Could you check a few things on this model? Use its own coordinates, in mm. Face numbers are marked on the shaded views. A direction names the side the tool comes from. Give positions to 0.01 mm unless a question says otherwise; leave off trailing zeros. Write each loop counter-clockwise with the first axis right and the second up, starting at its lowest first coordinate (ties: lowest second). Pieces come first, ordered by that corner, then holes. Notation, with made-up numbers: (67.5, 79.25) - (125.5, 79.25) arc R27 cw to (125.5, 117.25) - close; hole circle Ø7 at (4, 23.25). An arc over 180 degrees is marked (long way). Answer in a Markdown table with one row per item.
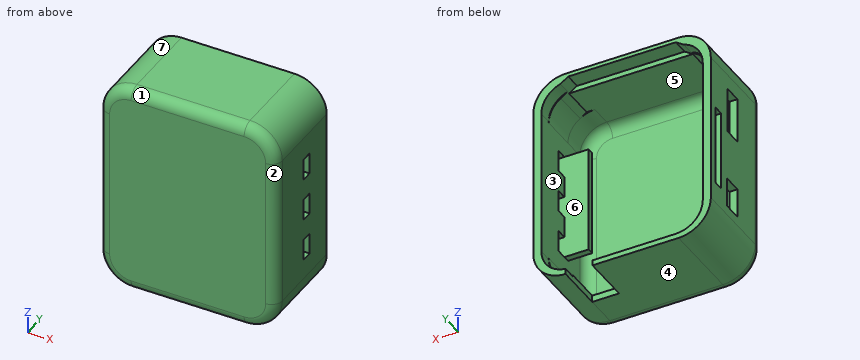
from build123d import *

# Parameters (mm, degrees)
EXTRUDE_1_DEPTH     = 9
EXTRUDE_2_DEPTH     = 1
SKETCH_4_W          = 8.5
SKETCH_4_H          = 3.4
SKETCH_4_W_2        = 15
SKETCH_4_H_2        = 2
SKETCH_4_W_3        = 5.5
SKETCH_4_H_3        = 3.5
CUT_EXTRUDE_1_DEPTH = 21
CUT_EXTRUDE_2_DEPTH = 7
EXTRUDE_3_DEPTH     = 6
SKETCH_9_W          = 5
SKETCH_9_H          = 1.5
CUT_EXTRUDE_4_DEPTH = 9
SKETCH_10_W         = 4.5
SKETCH_10_H         = 20
EXTRUDE_4_DEPTH     = 1.2
CUT_EXTRUDE_5_DEPTH = 2.5
CUT_EXTRUDE_6_DEPTH = 10
EXTRUDE_5_DEPTH     = 6
EXTRUDE_6_DEPTH     = 2
FILLET_1_R          = 2


with BuildPart() as part:
    # Sketch 1 → Extrude 1 (new body)
    with BuildSketch(Plane(origin=(0, 0, 0), x_dir=(1, 0, 0), z_dir=(0, 1, 0))):
        with BuildLine():
            Line((-15, -13.5), (-15, 0))
            Line((-15, 0), (-16.5, 0))
            Line((-16.5, 0), (-16.5, -14.25))
            ThreePointArc((-16.5, -14.25), (-14.742640687, -18.492640687), (-10.5, -20.25))
            Line((-10.5, -20.25), (0, -20.25))
            Line((0, -20.25), (0, -19.500334285))
            Line((0, -19.500334285), (-10, -19.500334285))
            Line((-10, -19.500334285), (-12.764203909, -17.666434537))
            ThreePointArc((-12.764203909, -17.666434537), (-14.405736008, -15.864210276), (-15, -13.5))
        make_face()
        with BuildLine():
            Line((16.5, 0), (15, 0))
            Line((15, 0), (15, -13.5))
            ThreePointArc((15, -13.5), (14.405736008, -15.864210276), (12.764203909, -17.666434537))
            Line((12.764203909, -17.666434537), (10, -19.500334285))
            Line((10, -19.500334285), (0, -19.500334285))
            Line((0, -19.500334285), (0, -20.25))
            Line((0, -20.25), (10.5, -20.25))
            ThreePointArc((10.5, -20.25), (14.742640687, -18.492640687), (16.5, -14.25))
            Line((16.5, -14.25), (16.5, 0))
        make_face()
        with BuildLine():
            Line((0, 19.75), (0, 18.5))
            Line((0, 18.5), (10, 18.5))
            ThreePointArc((10, 18.5), (13.535533906, 17.035533906), (15, 13.5))
            Line((15, 13.5), (15, 0))
            Line((15, 0), (16.5, 0))
            Line((16.5, 0), (16.5, 13.75))
            ThreePointArc((16.5, 13.75), (14.742640687, 17.992640687), (10.5, 19.75))
            Line((10.5, 19.75), (0, 19.75))
        make_face()
        with BuildLine():
            Line((-10, 18.5), (0, 18.5))
            Line((0, 18.5), (0, 19.75))
            Line((0, 19.75), (-10.5, 19.75))
            ThreePointArc((-10.5, 19.75), (-14.742640687, 17.992640687), (-16.5, 13.75))
            Line((-16.5, 13.75), (-16.5, 0))
            Line((-16.5, 0), (-15, 0))
            Line((-15, 0), (-15, 13.5))
            ThreePointArc((-15, 13.5), (-13.535533906, 17.035533906), (-10, 18.5))
        make_face()
    extrude(amount=-EXTRUDE_1_DEPTH)

    # Sketch 3 → Extrude 2 (add)
    with BuildSketch(Plane.XZ.offset(9)):
        with BuildLine():
            Line((-10.5, -19.75), (10.5, -19.75))
            ThreePointArc((10.5, -19.75), (14.742640687, -17.992640687), (16.5, -13.75))
            Line((16.5, -13.75), (16.5, 14.25))
            ThreePointArc((16.5, 14.25), (14.742640687, 18.492640687), (10.5, 20.25))
            Line((10.5, 20.25), (-10.5, 20.25))
            ThreePointArc((-10.5, 20.25), (-14.742640687, 18.492640687), (-16.5, 14.25))
            Line((-16.5, 14.25), (-16.5, -13.75))
            ThreePointArc((-16.5, -13.75), (-14.742640687, -17.992640687), (-10.5, -19.75))
        make_face()
    extrude(amount=EXTRUDE_2_DEPTH)

    # Sketch 4 → Cut-Extrude 1 (cut)
    with BuildSketch(Plane(origin=(-15, 0, 0), x_dir=(0, 0, -1), z_dir=(1, 0, 0))):
        with Locations((-7.250334285, -7.3)):
            Rectangle(SKETCH_4_W, SKETCH_4_H)
        with Locations((2.25, -2.5)):
            Rectangle(SKETCH_4_W_2, SKETCH_4_H_2)
        with Locations((9.25, -7.25)):
            Rectangle(SKETCH_4_W_3, SKETCH_4_H_3)
    extrude(amount=-CUT_EXTRUDE_1_DEPTH, mode=Mode.SUBTRACT)

    # Sketch 5 → Cut-Extrude 2 (cut)
    with BuildSketch(Plane.ZY.offset(-15)):
        Polygon((-2, -5.8), (-2, -7.8), (0, -7.8), (2, -7.8), (2, -5.8), align=None)
        Polygon((10, -7.8), (8, -7.8), (6, -7.8), (6, -5.8), (10, -5.8), align=None)
        Polygon((-10, -5.8), (-10, -7.8), (-8, -7.8), (-6, -7.8), (-6, -5.8), align=None)
    extrude(amount=-CUT_EXTRUDE_2_DEPTH, mode=Mode.SUBTRACT)

    # Sketch 6 → Extrude 3 (add)
    with BuildSketch(Plane(origin=(0, -9, 0), x_dir=(1, 0, 0), z_dir=(0, 1, 0))):
        Polygon((10, -19.500334285), (11.507785769, -18.5), (10, -18.5), (-10, -18.5), (-11.507785769, -18.5), (-10, -19.500334285), align=None)
    extrude(amount=EXTRUDE_3_DEPTH)

    # Sketch 9 → Cut-Extrude 4 (cut)
    with BuildSketch(Plane(origin=(0, 0, 0), x_dir=(1, 0, 0), z_dir=(0, 1, 0))):
        with Locations((8, 19)):
            Rectangle(SKETCH_9_W, SKETCH_9_H)
    extrude(amount=-CUT_EXTRUDE_4_DEPTH, mode=Mode.SUBTRACT)

    # Sketch 10 → Extrude 4 (add)
    with BuildSketch(Plane(origin=(0, -9, 0), x_dir=(1, 0, 0), z_dir=(0, 1, 0))):
        with Locations((12.75, 0)):
            Rectangle(SKETCH_10_W, SKETCH_10_H)
    extrude(amount=EXTRUDE_4_DEPTH)

    # Sketch 12 → Cut-Extrude 5 (cut)
    with BuildSketch(Plane(origin=(0, 0, 0), x_dir=(1, 0, 0), z_dir=(0, 1, 0))):
        with BuildLine():
            Line((10, -18.75), (-10, -18.75))
            ThreePointArc((-10, -18.75), (-13.535533906, -17.285533906), (-15, -13.75))
            Line((-15, -13.75), (-15, 13.75))
            ThreePointArc((-15, 13.75), (-13.535533906, 17.285533906), (-10, 18.75))
            Line((-10, 18.75), (10, 18.75))
            ThreePointArc((10, 18.75), (13.535533906, 17.285533906), (15, 13.75))
            Line((15, 13.75), (15, -13.75))
            ThreePointArc((15, -13.75), (13.535533906, -17.285533906), (10, -18.75))
        make_face()
    extrude(amount=-CUT_EXTRUDE_5_DEPTH, mode=Mode.SUBTRACT)

    # Sketch 13 → Cut-Extrude 6 (cut)
    with BuildSketch(Plane(origin=(0, -9, 0), x_dir=(1, 0, 0), z_dir=(0, 1, 0))):
        with BuildLine():
            Line((-10, -18.5), (10, -18.5))
            ThreePointArc((10, -18.5), (13.535533906, -17.035533906), (15, -13.5))
            Line((15, -13.5), (15, 13.5))
            ThreePointArc((15, 13.5), (13.535533906, 17.035533906), (10, 18.5))
            Line((10, 18.5), (-10, 18.5))
            ThreePointArc((-10, 18.5), (-13.535533906, 17.035533906), (-15, 13.5))
            Line((-15, 13.5), (-15, -13.5))
            ThreePointArc((-15, -13.5), (-13.535533906, -17.035533906), (-10, -18.5))
        make_face()
    extrude(amount=-CUT_EXTRUDE_6_DEPTH, mode=Mode.SUBTRACT)

    # Sketch 14 → Extrude 5 (add)
    with BuildSketch(Plane.XZ.offset(9)):
        with BuildLine():
            Line((-10.5, -19.75), (10.5, -19.75))
            ThreePointArc((10.5, -19.75), (14.742640687, -17.992640687), (16.5, -13.75))
            Line((16.5, -13.75), (16.5, 14.25))
            ThreePointArc((16.5, 14.25), (14.742640687, 18.492640687), (10.5, 20.25))
            Line((10.5, 20.25), (-10.5, 20.25))
            ThreePointArc((-10.5, 20.25), (-14.742640687, 18.492640687), (-16.5, 14.25))
            Line((-16.5, 14.25), (-16.5, -13.75))
            ThreePointArc((-16.5, -13.75), (-14.742640687, -17.992640687), (-10.5, -19.75))
        make_face()
        with BuildLine():
            Line((-10, -18.5), (10, -18.5))
            ThreePointArc((10, -18.5), (13.535533906, -17.035533906), (15, -13.5))
            Line((15, -13.5), (15, 13.5))
            ThreePointArc((15, 13.5), (13.535533906, 17.035533906), (10, 18.5))
            Line((10, 18.5), (-10, 18.5))
            ThreePointArc((-10, 18.5), (-13.535533906, 17.035533906), (-15, 13.5))
            Line((-15, 13.5), (-15, -13.5))
            ThreePointArc((-15, -13.5), (-13.535533906, -17.035533906), (-10, -18.5))
        make_face(mode=Mode.SUBTRACT)
    extrude(amount=EXTRUDE_5_DEPTH)

    # Sketch 15 → Extrude 6 (add)
    with BuildSketch(Plane.XZ.offset(15)):
        with BuildLine():
            Line((-10.5, 20.25), (10.5, 20.25))
            ThreePointArc((10.5, 20.25), (14.742640687, 18.492640687), (16.5, 14.25))
            Line((16.5, 14.25), (16.5, -13.75))
            ThreePointArc((16.5, -13.75), (14.742640687, -17.992640687), (10.5, -19.75))
            Line((10.5, -19.75), (-10.5, -19.75))
            ThreePointArc((-10.5, -19.75), (-14.742640687, -17.992640687), (-16.5, -13.75))
            Line((-16.5, -13.75), (-16.5, 14.25))
            ThreePointArc((-16.5, 14.25), (-14.742640687, 18.492640687), (-10.5, 20.25))
        make_face()
    extrude(amount=EXTRUDE_6_DEPTH)

    # Fillet 1
    fillet_1_edges = [part.edges().sort_by_distance(p)[0] for p in [
        (13.535533906, -15, -17.035533906),
        (0, -15, -18.5),
        (13.535533906, -15, 17.035533906),
        (15, -15, 0),
        (-13.535533906, -15, 17.035533906),
        (0, -15, 18.5),
        (-13.535533906, -15, -17.035533906),
        (-15, -15, 0),
        (-14.742640687, -17, -17.992640687),
        (0, -17, -19.75),
        (14.742640687, -17, -17.992640687),
        (16.5, -17, 0.25),
        (14.742640687, -17, 18.492640687),
        (0, -17, 20.25),
        (-14.742640687, -17, 18.492640687),
        (-16.5, -17, 0.25),
    ]]
    fillet(fillet_1_edges, radius=FILLET_1_R)


solid = part.part
1) We'd pull the mould along Z, two halves only. Please class the marked faces 1, 2, 3 and 4: +Z half, -Z half, draft (parallel to the pull), parting line (faces both ways), or undercut.
Check values:
| item | result |
|---|---|
| face 1 | +Z half |
| face 2 | draft |
| face 3 | undercut |
| face 4 | -Z half |
2) On a 3-axis mill with a long thin cutter (end or side, diameter ignored), from which of +Z, -Z, +X, -X, +Y, -Y can I reach the whole of each face in a straight line? I mean the marked faces 5, 6 and 7. Say none if no direction works.
Check values:
| item | result |
|---|---|
| face 5 | +Y |
| face 6 | none |
| face 7 | +Z, -X, +Y, -Y |
3) If I drill on line 1 (X direction, y = -5.25, z = 4.5); line 2 (Z direction, x = 1, y = -2.25); line 3 (Z direction, x = 0.5, y = -7), over which ranges is the centre line in solid material (lowest first)?
Check values:
| item | result |
|---|---|
| line 1 | x = -16.5 to -15, 15 to 16.5 |
| line 2 | z = -19.75 to -18.75, 19.5 to 20.25 |
| line 3 | z = -19.75 to -18.5, 18.5 to 20.25 |
4) Imagine slicing it at C-C (z = -4). List the corners of the cut face in (x, y) for me, then the cut area to 3 significant figures.
Check values:
| item | result |
|---|---|
| outline | (-16.5, -15) arc R2 ccw to (-14.5, -17) - (14.5, -17) arc R2 ccw to (16.5, -15) - (16.5, 0) - (15, 0) - (15, -7.8) - (10.5, -7.8) - (10.5, -9) - (15, -9) - (15, -13) arc R2 cw to (13, -15) - (-13, -15) arc R2 cw to (-15, -13) - (-15, -3.5) - (-16.5, -3.5) - close; (-16.5, -1.5) - (-15, -1.5) - (-15, 0) - (-16.5, 0) - close |
| area | 113 mm2 |
5) Will these pins go through, and if not, where does the flat tip stop? P1, Ø3, axis at x = 14.5, z = 2.5, coming from the +Y side; P2, Ø0.6, axis at x = 7, z = -19, coming from the +Y side; P3, Ø1, axis at y = -2.5, z = -19, coming from the -X side; P4, Ø1.2, axis at x = -16, y = -6.5, coming from the -Z side.
Check values:
| item | result |
|---|---|
| P1 | stops at y = 0 |
| P2 | stops at y = -9 |
| P3 | stops at x = -14.17 |
| P4 | stops at z = -17.21 |
6) Imagine slicing it at D-D (x = -1). List the corners of the cut face in (y, z) for me, then the cut area to 3 significant figures.
Check values:
| item | result |
|---|---|
| outline | (-17, -17.75) arc R2 ccw to (-15, -19.75) - (0, -19.75) - (0, -18.75) - (-2.5, -18.75) - (-2.5, -18.5) - (-13, -18.5) arc R2 cw to (-15, -16.5) - (-15, 16.5) arc R2 cw to (-13, 18.5) - (-3, 18.5) - (-3, 19.5) - (0, 19.5) - (0, 20.25) - (-15, 20.25) arc R2 ccw to (-17, 18.25) - close |
| area | 121 mm2 |
7) Imagine slicing it at B-B (y = -12). List the corners of the cut face in (x, z) for me.
Check values:
| item | result |
|---|---|
| outline | (-16.5, -13.75) arc R6 ccw to (-10.5, -19.75) - (10.5, -19.75) arc R6 ccw to (16.5, -13.75) - (16.5, 14.25) arc R6 ccw to (10.5, 20.25) - (-10.5, 20.25) arc R6 ccw to (-16.5, 14.25) - close; hole (-15, -13.5) arc R5 ccw to (-10, -18.5) - (10, -18.5) arc R5 ccw to (15, -13.5) - (15, 13.5) arc R5 ccw to (10, 18.5) - (-10, 18.5) arc R5 ccw to (-15, 13.5) - close |
8) Imagine slicing it at A-A (z = -8). List the corners of the cut face in (x, y) for me.
Check values:
| item | result |
|---|---|
| outline | (-16.5, -15) arc R2 ccw to (-14.5, -17) - (14.5, -17) arc R2 ccw to (16.5, -15) - (16.5, -7.8) - (10.5, -7.8) - (10.5, -9) - (15, -9) - (15, -13) arc R2 cw to (13, -15) - (-13, -15) arc R2 cw to (-15, -13) - (-15, -9) - (-16.5, -9) - close; (-16.5, -5.5) - (-15, -5.5) - (-15, -3.5) - (-16.5, -3.5) - close; (-16.5, -1.5) - (-15, -1.5) - (-15, 0) - (-16.5, 0) - close; (15, -5.8) - (16.5, -5.8) - (16.5, 0) - (15, 0) - close |
